from build123d import *

# Parameters (mm, degrees)
F1_DEPTH  = 252
F4_DEPTH  = 20
F6_DEPTH  = 50.001
F7_R      = 5
F8_R      = 5
F9_W      = 180
F9_H      = 217
F10_DEPTH = 25
F11_R     = 10


with BuildPart() as f1:
    # F0 (on Front) → F1 (new body)
    with BuildSketch(Plane.XZ):
        Polygon((100, 0), (0, 0), (0, -50), (65.3589838486, -50), (100, -30), align=None)
    extrude(amount=F1_DEPTH)

    # F2: F1 across plane


with BuildPart() as f1_1:
    add(f1.part)
    add(f1.part.mirror(Plane.YZ))

    # F3 (on face) → F4 (cut)
    with BuildSketch(Plane.XY):
        Polygon((-60, -252), (60, -252), (60, -50), (0, -128.1935223705), (-60, -50), align=None)
    extrude(amount=-F4_DEPTH, mode=Mode.SUBTRACT)

    # F5 (on face) → F6 (cut, through all)
    with BuildSketch(Plane.XY):
        with BuildLine():
            ThreePointArc((100, -212), (88.2842712475, -240.2842712475), (60, -252))
            Line((60, -252), (100, -252))
            Line((100, -252), (100, -212))
        make_face()
        with BuildLine():
            Line((-100, -252), (-60, -252))
            ThreePointArc((-60, -252), (-88.2842712475, -240.2842712475), (-100, -212))
            Line((-100, -212), (-100, -252))
        make_face()
    extrude(amount=-F6_DEPTH, mode=Mode.SUBTRACT)

    # F7
    f7_edges = [f1_1.edges().sort_by_distance(p)[0] for p in [
        (0, -128.193522, -10),
    ]]
    fillet(f7_edges, radius=F7_R)

    # F8
    f8_edges = [f1_1.edges().sort_by_distance(p)[0] for p in [
        (60, -50, -10),
        (-60, -50, -10),
    ]]
    fillet(f8_edges, radius=F8_R)

    # F9 (on face) → F10 (cut)
    with BuildSketch(Plane(origin=(0, 0, -50), x_dir=(1, 0, 0), z_dir=(0, 0, -1))):
        with Locations((0, 118.5)):
            Rectangle(F9_W, F9_H)
    extrude(amount=-F10_DEPTH, mode=Mode.SUBTRACT)

    # F11
    f11_edges = [f1_1.edges().sort_by_distance(p)[0] for p in [
        (90, -10, -30.386751),
        (-90, -10, -30.386751),
        (-90, -227, -30.386751),
        (90, -227, -30.386751),
    ]]
    fillet(f11_edges, radius=F11_R)


solid = f1_1.part
Part model, mm, in its own coordinate system. A direction names the side the tool comes from. Give positions to 0.01 mm unless a question says otherwise; leave off trailing zeros. Order: outer loops, then holes, each group sorted by start corner. A loop starts at its lowest first (then second) coordinate and runs counter-clockwise, first axis right, second up. Notation, with made-up numbers: (-34.5, 7) - (-24.5, 7) arc R24 cw to (-24.5, 29) - close; hole circle Ø4 at (87, -32). An arc over 180 degrees is marked (long way). Use a Markdown table: item, result.
1) Saw through at A-A on y = -185.5. List the corners of the cut face in (x, z), plus the area to 3 significant figures.
Checked values:
| item | result |
|---|---|
| outline | (-100, -30) - (-90, -35.77) - (-90, -25) - (90, -25) - (90, -35.77) - (100, -30) - (100, 0) - (60, 0) - (60, -20) - (-60, -20) - (-60, 0) - (-100, 0) - close |
| area | 2,760 mm² |
2) Saw through at D-D on y = -40.5. List the corners of the cut face in (x, z), plus the area to 3 significant figures.
Checked values:
| item | result |
|---|---|
| outline | (-100, -30) - (-90, -35.77) - (-90, -25) - (90, -25) - (90, -35.77) - (100, -30) - (100, 0) - (-100, 0) - close |
| area | 5,160 mm² |
3) Probe L1, parallel to X at y = -118.5, z = -3; L2, parallel to Y at x = -33.5, z = -34; L3, parallel to X at y = -113, z = -27. List the from-to ranges inside material, lowest first. Write a range as from..to.
Checked values:
| item | result |
|---|---|
| L1 | -100..-60, -7.44..7.44, 60..100 |
| L2 | -252..-227, -10..0 |
| L3 | -100..-90, 90..100 |
4) 3-axis set-ups, long thin cutter, end or side, ignore diameter. For faces 1 (the flat face through (-1, -96, 0)), 2 (the flat face through (-1, -120, -25)), 3 (the flat face through (-60, -157, -10)): which of +Z, -Z, +X, -X, +Y, -Y reach the whole face in a straight line?
Checked values:
| item | result |
|---|---|
| face 1 | +Z, +X, -X, +Y, -Y |
| face 2 | -Z |
| face 3 | +Z, -Y |
5) Two-plate mould, pull along X, no slides. Class faces 4 (the flat face through (-93.984, -124.058, -33.473)), 5 (the flat face through (100, -105, -15)), 6 (the cylindrical face through (86.99, -224.15, -31.32)): +X half, -X half, draft (parallel to the pull), parting line (faces both ways), or undercut.
Checked values:
| item | result |
|---|---|
| face 4 | -X half |
| face 5 | +X half |
| face 6 | undercut |
6) Saw through at C-C on x = 15.5. List the corners of the cut face in (y, z).
Checked values:
| item | result |
|---|---|
| outline | (-252, -50) - (-227, -50) - (-227, -25) - (-10, -25) - (-10, -50) - (0, -50) - (0, 0) - (-107.99, 0) - (-107.99, -20) - (-252, -20) - close |
7) Saw through at B-B on z = -13.5. List the corners of the cut face in (x, y), plus the area to 3 significant figures.
Checked values:
| item | result |
|---|---|
| outline | (-100, -212) arc R40 ccw to (-60, -252) - (-60, -64.73) arc R5 cw to (-51.03, -61.69) - (-3.97, -123.02) arc R5 ccw to (3.97, -123.02) - (51.03, -61.69) arc R5 cw to (60, -64.73) - (60, -252) arc R40 ccw to (100, -212) - (100, 0) - (-100, 0) - close |
| area | 30,200 mm² |
8) Flat gauge pins, fed straight in: P1, Ø8, axis at x = 40, y = -178.5, coming from the -Z side; P2, Ø1.5, axis at x = -62, z = -38.5, coming from the -Y side; P3, Ø8, axis at x = -28.5, y = -210, coming from the +Z side. Where does each tip first touch, or does it go through?
Checked values:
| item | result |
|---|---|
| P1 | z = -25 |
| P2 | y = -251.98 |
| P3 | z = -20 |
